Input: part model. Units: mm. Frame: model coordinates. Give positions to 0.01 mm unless a question says otherwise; leave off trailing zeros. Write each loop counter-clockwise with the first axis right and the second up, starting at its lowest first coordinate (ties: lowest second). Pieces come first, ordered by that corner, then holes. Notation, with made-up numbers: (-10.75, -7.5) - (21.25, -7.5) arc R27 ccw to (21.25, 31.5) - close; hole circle Ø1 at (87.25, 34.25). An arc over 180 degrees is marked (long way). Answer as CSV lines item,"result". Start each with the question number.
from build123d import *

# Parameters (mm, degrees)
SKETCH1_R           = 2.25
BOSS_EXTRUDE1_DEPTH = 4.7625


with BuildPart() as part:
    # Sketch1 → Boss-Extrude1 (new body)
    # profile 1 of 3: a face of its own
    with BuildSketch(Plane.XY):
        with BuildLine():
            Line((-3.5, 27.5), (-3.5, -7.5))
            Line((-3.5, -7.5), (35.5, -7.5))
            Line((35.5, -7.5), (35.5, 27.5))
            Line((35.5, 27.5), (35.5, 47.5))
            Line((35.5, 47.5), (28.5, 47.5))
            Line((28.5, 47.5), (28.5, 37.5))
            ThreePointArc((28.5, 37.5), (26, 35), (23.5, 37.5))
            Line((23.5, 37.5), (23.5, 47.5))
            Line((23.5, 47.5), (8.5, 47.5))
            Line((8.5, 47.5), (8.5, 37.5))
            ThreePointArc((8.5, 37.5), (6, 35), (3.5, 37.5))
            Line((3.5, 37.5), (3.5, 47.5))
            Line((3.5, 47.5), (-3.5, 47.5))
            Line((-3.5, 47.5), (-3.5, 27.5))
        make_face()
        with Locations(Location((0, 0, 0), (0, 0, 180))):
            Circle(SKETCH1_R, mode=Mode.SUBTRACT)
        with Locations(Location((0, 20, 0), (0, 0, 180))):
            Circle(SKETCH1_R, mode=Mode.SUBTRACT)
        with Locations(Location((32, 0, 0), (0, 0, 180))):
            Circle(SKETCH1_R, mode=Mode.SUBTRACT)
        with Locations(Location((32, 20, 0), (0, 0, 180))):
            Circle(SKETCH1_R, mode=Mode.SUBTRACT)
    # profile 2 of 3: a face of its own
    with BuildSketch(Plane.XY):
        with BuildLine():
            Line((8.5, 47.5), (3.5, 47.5))
            Line((3.5, 47.5), (3.5, 37.5))
            ThreePointArc((3.5, 37.5), (6, 40), (8.5, 37.5))
            Line((8.5, 37.5), (8.5, 47.5))
        make_face()
    # profile 3 of 3: a face of its own
    with BuildSketch(Plane.XY):
        with BuildLine():
            Line((28.5, 37.5), (28.5, 47.5))
            Line((28.5, 47.5), (23.5, 47.5))
            Line((23.5, 47.5), (23.5, 37.5))
            ThreePointArc((23.5, 37.5), (26, 40), (28.5, 37.5))
        make_face()
    extrude(amount=BOSS_EXTRUDE1_DEPTH)


solid = part.part
1) Pull-direction query (X, two-part tool) for faces 1 (the flat face through (16, -7.5, 2)), 2 (the flat face through (-3.5, 20, 2)), 3 (the flat face through (35.5, 20, 2)), 4 (the cylindrical face through (1.66, -1.52, 2.35)); classes: +X half, -X half, draft (parallel to the pull), parting line (faces both ways), or undercut.
2) Cut plane A-A on x = 32. Output: boundary loops of the cut face in (y, z), and give its area (3 significant figures).
3) Cut plane C-C on x = 26. Output: boundary loops of the cut face in (y, z).
4) Cut plane D-D on z = 1.5. Output: boundary loops of the cut face in (x, y), and give its area (3 significant figures).
5) Cut plane B-B on y = 37.5. Output: boundary loops of the cut face in (x, z), and give its area (3 significant figures).
6) Material intervals for line 1 (Y direction, x = 32, z = 3.35); line 2 (X direction, y = 37.5, z = 1.95); line 3 (X direction, y = 37, z = 2.6), sorted ascending. Write a range as from..to.
Numbers:
1,face 1,"draft"
1,face 2,"-X half"
1,face 3,"+X half"
1,face 4,"undercut"
2,outline,"(-7.5, 0) - (-2.25, 0) - (-2.25, 4.76) - (-7.5, 4.76) - close; (2.25, 0) - (17.75, 0) - (17.75, 4.76) - (2.25, 4.76) - close; (22.25, 0) - (47.5, 0) - (47.5, 4.76) - (22.25, 4.76) - close"
2,area,"219 mm²"
3,outline,"(-7.5, 0) - (35, 0) - (35, 4.76) - (-7.5, 4.76) - close; (40, 0) - (47.5, 0) - (47.5, 4.76) - (40, 4.76) - close"
4,outline,"(-3.5, -7.5) - (35.5, -7.5) - (35.5, 47.5) - (-3.5, 47.5) - close; hole circle Ø4.5 at (0, 0); hole circle Ø4.5 at (0, 20); hole circle Ø5 at (6, 37.5); hole circle Ø5 at (26, 37.5); hole circle Ø4.5 at (32, 0); hole circle Ø4.5 at (32, 20)"
4,area,"2,040 mm²"
5,outline,"(-3.5, 0) - (3.5, 0) - (3.5, 4.76) - (-3.5, 4.76) - close; (8.5, 0) - (23.5, 0) - (23.5, 4.76) - (8.5, 4.76) - close; (28.5, 0) - (35.5, 0) - (35.5, 4.76) - (28.5, 4.76) - close"
5,area,"138 mm²"
6,line 1,"y = -7.5..-2.25, 2.25..17.75, 22.25..47.5"
6,line 2,"x = -3.5..3.5, 8.5..23.5, 28.5..35.5"
6,line 3,"x = -3.5..3.55, 8.45..23.55, 28.45..35.5"
